Here's how the part is built. I have some questions about the finished solid (model axes, mm). A direction names the side the tool comes from. Coordinates: 2 decimals unless noted, no trailing zeros. Write each loop counter-clockwise with the first axis right and the second up, starting at its lowest first coordinate (ties: lowest second). Pieces come first, ordered by that corner, then holes. Notation, with made-up numbers: (58, 40) -> (112, 40) arc R25 cw to (112, 53) -> close; hole circle Ø6 at (-5.5, -17.5). An arc over 180 degrees is marked (long way). Use CSV: the item, a comma, the result in double quotes. Start each with the question number.
```python
from build123d import *

# Parameters (mm, degrees)
KES_EKSTR_ZYON1_DEPTH = 18


with BuildPart() as part:
    # Çizim1 → Döndür3 (revolve)
    with BuildSketch(Plane.XY):
        with BuildLine():
            Line((-1.32512155, 2.139611708), (-1.32512155, 0.570301782))
            Line((-1.32512155, 0.570301782), (-0.411194993, 0.570301782))
            ThreePointArc((-0.411194993, 0.570301782), (-0.422380451, 0.285248389), (-0.426109787, 0))
            Line((-0.426109787, 0), (0, 0))
            ThreePointArc((0, 0), (1.957189595, 6.100058308), (7.098060997, 9.922720168))
            Line((7.098060997, 9.922720168), (7.098060997, 10.723199249))
            ThreePointArc((7.098060997, 10.723199249), (2.598216191, 8.016184499), (-0.181803757, 3.56107269))
            ThreePointArc((-0.181803757, 3.56107269), (-0.35786127, 3.666258696), (-0.558844205, 3.707077853))
            Line((-0.558844205, 3.707077853), (-5.367482514, 3.707077853))
            Line((-5.367482514, 3.707077853), (-6.581672956, 2.928819663))
            Line((-6.581672956, 2.928819663), (-6.581672956, 2.145222918))
            Line((-6.581672956, 2.145222918), (-1.32512155, 2.139611708))
        make_face()
    revolve(axis=Axis((0, 0, 0), (-1, 0, 0)))

    # Çizim2 → Kes-Ekstrüzyon1 (cut)
    with BuildSketch(Plane.ZY.offset(6.581672956)):
        Polygon((-4.065, 0), (-4.065, 9.922841183), (-12.277622452, 10.110434639), (-12.277622452, -10.854234794), (-4.065, -10.854234794), align=None)
        Polygon((4.065, 0), (4.065, 10.512736346), (12.14810156, 10.512736346), (12.606032623, -11.349214468), (4.065, -11.349214468), align=None)
    extrude(amount=-KES_EKSTR_ZYON1_DEPTH, mode=Mode.SUBTRACT)


solid = part.part
```
Item 1: I want a section at D-D on x = -4.25. Please give me the cut outline in (y, z).
Item 2: Which directions (+Z, -Z, +X, -X, +Y, -Y) give clear straight access to the entire face, cutting with the end or side of a thin tool? Please do faces 1 (the cylindrical face through (-0.862, 0.544, -0.171)), 2 (the flat face through (0.6, 0, 4.065)).
Item 3: If I drill on line 1 along Z through (x, y) = (-0.9, 0); line 2 along Y through (x, z) = (6, 1.25), over which ranges is the centre line in solid material (lowest first)?
Item 4: I'm going to push flat-ended pins straight in: pin 1 (1 mm diameter, centred on y = 0, z = 0, fed in from -X); pin 2 (3 mm diameter, centred on y = -7.5, z = 2, fed in from +X); pin 3 (1.5 mm diameter, centred on y = -5.5, z = -3, fed in from -X). Where does each tip first touch, or does it pass through?
Item 5: I want a section at B-B on x = -1.75. Please give me the cut outline in (y, z).
Item 6: Thinking about a two-plate mould opening in Z: for faces 3 (the conical face through (-3.917, 2.043, -0.644)), 4 (the cylindrical face through (-2.997, 3.536, -1.114)), 5 (the flat face through (7.098, -10.1, -0.1)), which applies, +Z half, -Z half, draft (parallel to the pull), parting line (faces both ways), or undercut?
Item 7: I want a section at C-C on y = 5.5. Please give me the cut outline in (x, z) (1 decimal), then the cut area to 3 significant figures.
Item 8: I want a section at A-A on x = 4.25. Please give me the cut outline in (y, z) (3 decimals).
Geometry says:
1,outline,"circle Ø7.41 at (0, 0); hole circle Ø4.29 at (0, 0)"
2,face 1,"-X"
2,face 2,"+Z, +X, -X, +Y, -Y"
3,line 1,"-3.71 to -0.57, 0.57 to 3.71"
3,line 2,"-10.24 to -9.39, 9.39 to 10.24"
4,pin 1,"x = -0.43"
4,pin 2,"x = 5.57"
4,pin 3,"x = 0.68"
5,outline,"circle Ø7.41 at (0, 0); hole circle Ø4.28 at (0, 0)"
6,face 3,"undercut"
6,face 4,"parting line"
6,face 5,"draft"
7,outline,"(1.6, -4.1) -> (2.5, -4.1) arc R8.9 cw to (2.5, 4.1) -> (1.6, 4.1) arc R9.8 ccw to start"
7,area,"7.42 mm2"
8,outline,"(-8.43, -4.065) -> (-7.385, -4.065) arc R8.43 cw to (-7.385, 4.065) -> (-8.43, 4.065) arc R9.359 ccw to start; (7.385, -4.065) -> (8.43, -4.065) arc R9.359 ccw to (8.43, 4.065) -> (7.385, 4.065) arc R8.43 cw to start"
